CAD build for the part. Positions are in the model's coordinates, mm. A direction names the side the tool comes from. Round coordinates to 2 decimals unless told otherwise and drop trailing zeros. Order: outer loops, then holes, each group sorted by start corner. A loop starts at its lowest first (then second) coordinate and runs counter-clockwise, first axis right, second up.
```python
from build123d import *

# Parameters (mm, degrees)
BOSS_EXTRUDE1_DEPTH = 9
SKETCH2_W           = 74.887018594
SKETCH2_H           = 25.704308128
CUT_EXTRUDE1_DEPTH  = 10
SKETCH3_W           = 13
SKETCH3_H           = 19
CUT_EXTRUDE2_DEPTH  = 10
SKETCH4_W           = 180
SKETCH4_H           = 55
CUT_EXTRUDE3_DEPTH  = 478.310586352


with BuildPart() as part:
    # Sketch1 → Boss-Extrude1 (new body)
    with BuildSketch(Plane.XY):
        Polygon((169.032702555, 364.5), (109.032702555, 364.5), (109.032702555, 355.5), (49.032702555, 355.5), (49.032702555, 364.5), (-20.967297445, 364.5), (-20.967297445, 270.5), (-29.967297445, 270.5), (-29.967297445, 210.5), (-20.967297445, 210.5), (-20.967297445, 150.5), (-29.967297445, 150.5), (-29.967297445, 90.5), (-20.967297445, 90.5), (-20.967297445, -3.5), (49.032702555, -3.5), (49.032702555, 5.5), (109.032702555, 5.5), (109.032702555, -3.5), (169.032702555, -3.5), (169.032702555, 5.5), (229.032702555, 5.5), (229.032702555, -3.5), (299.032702555, -3.5), (299.032702555, 90.5), (308.032702555, 90.5), (308.032702555, 150.5), (299.032702555, 150.5), (299.032702555, 210.5), (308.032702555, 210.5), (308.032702555, 270.5), (299.032702555, 270.5), (299.032702555, 364.5), (229.032702555, 364.5), (229.032702555, 355.5), (169.032702555, 355.5), align=None)
    extrude(amount=BOSS_EXTRUDE1_DEPTH)

    # Sketch2 → Cut-Extrude1 (cut)
    with BuildSketch(Plane(origin=(0, 0, 0), x_dir=(-1, 0, 0), z_dir=(0, 0, -1))):
        Polygon((20.967297445, 90.5), (-95.329165796, 90.5), (-95.329165796, 5.5), (9.317508813, 5.5), (29.967297445, 5.5), (29.967297445, 90.5), align=None)
        with Locations((-14.280157362, -7.352154064)):
            Rectangle(SKETCH2_W, SKETCH2_H)
    extrude(amount=-CUT_EXTRUDE1_DEPTH, mode=Mode.SUBTRACT)

    # Sketch3 → Cut-Extrude2 (cut)
    with BuildSketch(Plane(origin=(0, 0, 0), x_dir=(-1, 0, 0), z_dir=(0, 0, -1))):
        with Locations((-121.829165796, 45)):
            Rectangle(SKETCH3_W, SKETCH3_H)
    extrude(amount=-CUT_EXTRUDE2_DEPTH, mode=Mode.SUBTRACT)

    # Sketch4 → Cut-Extrude3 (cut, through all)
    with BuildSketch(Plane(origin=(0, 0, 0), x_dir=(-1, 0, 0), z_dir=(0, 0, -1))):
        with Locations((-139.032702555, 288)):
            Rectangle(SKETCH4_W, SKETCH4_H)
    extrude(amount=-CUT_EXTRUDE3_DEPTH, mode=Mode.SUBTRACT)


solid = part.part
```
1. Cut at A-A, the plane x = 213. Write the cut outline in (y, z).
2. Mould opens along X. For faces 1 (the face through (102, 5.5, 4)), 2 (the face through (128.329, 45, 4)), 3 (the face through (308.033, 120, 4)), 4 (the face through (115.329, 45, 4)) say: released by +X, released by -X, zero draft, split by the parting line, or undercut.
3. Cut at D-D, the plane z = 6.5. Give the number of separate pieces and of enclosed holes in the cut face, and give its area (3 significant figures).
4. Pin check, flat tips, straight feed: P1, Ø4.5, axis at x = 302, z = 4.5, coming from the +Y side; P2, Ø4.5, axis at y = 339.5, z = 3, coming from the -X side; P3, Ø2.5, axis at y = 330.5, z = 5, coming from the +X side. Stop position of each tip, or through.
5. Drill centre lines: line 1 (Y direction, x = 209, z = 8.75); line 2 (Y direction, x = 140.5, z = 3.25); line 3 (X direction, y = 46.5, z = 5.25). Where is each one in solid material? Low to high.
6. Cut at C-C, the plane x = 121. Write the cut outline in (y, z).
7. Cut at B-B, the plane y = 287. Write the cut outline in (x, z).
8. Tool access for faces 5 (the face through (199, 355.5, 4)), 6 (the face through (-20.967, 181, 4)), 7 (the face through (299.033, 43, 4)), 8 (the face through (299.033, 180, 4)), 9 (the face through (49.033, 288, 4)): list every direction of +Z, -Z, +X, -X, +Y, -Y with a clear straight run to the whole face (end or side of a thin tool).
Outcome:
1. outline: (5.5, 0) - (260.5, 0) - (260.5, 9) - (5.5, 9) - close; (315.5, 0) - (355.5, 0) - (355.5, 9) - (315.5, 9) - close
2. face 1: zero draft
2. face 2: undercut
2. face 3: released by +X
2. face 4: undercut
3. separate pieces: 1
3. enclosed holes: 2
3. area: 97,100 mm2
4. P1: stops at y = 270.5
4. P2: stops at x = -20.97
4. P3: stops at x = 299.03
5. line 1: y = 5.5 to 260.5, 315.5 to 355.5
5. line 2: y = -3.5 to 260.5, 315.5 to 364.5
5. line 3: x = 95.33 to 115.33, 128.33 to 299.03
6. outline: (-3.5, 0) - (35.5, 0) - (35.5, 9) - (-3.5, 9) - close; (54.5, 0) - (260.5, 0) - (260.5, 9) - (54.5, 9) - close; (315.5, 0) - (364.5, 0) - (364.5, 9) - (315.5, 9) - close
7. outline: (-20.97, 0) - (49.03, 0) - (49.03, 9) - (-20.97, 9) - close; (229.03, 0) - (299.03, 0) - (299.03, 9) - (229.03, 9) - close
8. face 5: +Z, -Z, +Y
8. face 6: +Z, -Z, -X
8. face 7: +Z, -Z, +X, -Y
8. face 8: +Z, -Z, +X
8. face 9: +Z, -Z
